Geometry: final body of the model. Coordinates: model frame, mm. Face numbers are marked on the shaded views. A direction names the side the tool comes from. Give positions to 0.01 mm unless a question says otherwise; leave off trailing zeros. Loops run counter-clockwise (first coordinate to the right, second up) from the corner with the lowest first, then second, coordinate; pieces in that order, holes last.
1. Section D-D, the plane x = -17.5. Output: boundary loops of the cut face in (y, z).
2. First-contact query: P1, Ø10, axis at y = -7.5, z = 57, coming from the +X side (3 decimals); P2, Ø2, axis at x = 8.5, z = -159.5, coming from the -Y side; P3, Ø10, axis at x = 20.5, z = 72, coming from the +Y side. Flat tips, straight axial feed; report the tip coordinate or a pass-through.
3. Section C-C, the plane x = 19. Output: boundary loops of the cut face in (y, z), then the cut area to 3 significant figures.
4. Access query for the marked faces 1, 2 and 3. Directions: +Z, -Z, +X, -X, +Y, -Y. A direction counts if a zero-diameter tool reaches every point of the face in a straight line with its end or side. Return the directions, or none.
5. Material intervals for line 1 along X through (y, z) = (-229.5, -87.5); line 2 along Z through (x, y) = (24, -132); line 3 along X through (y, z) = (-107, 112.5) (3 decimals), sorted ascending.
6. Draft query along Z for the marked faces 4 and 5. Return one class per face: +Z half, -Z half, draft (parallel to the pull), parting line (faces both ways), or undercut.
7. Section B-B, the plane y = 0. State how many separate pieces and enclosed holes the cut face has, then the cut area to 3 significant figures.
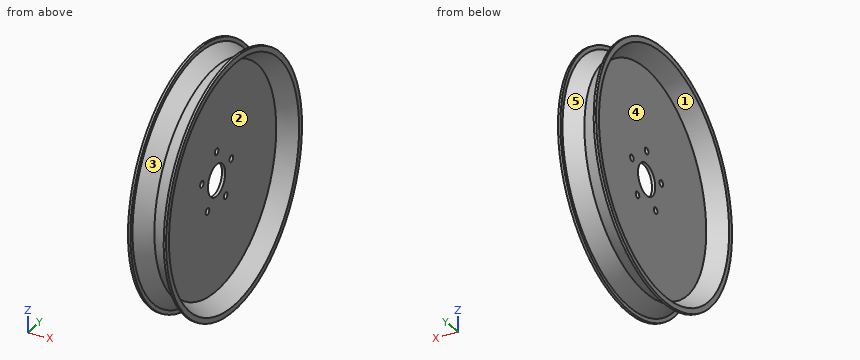
from build123d import *

# Parameters (mm, degrees)
F3_D = 13.1064


with BuildPart() as f1:
    # F0 (on Front) → F1 (revolve)
    with BuildSketch(Plane.XZ):
        Polygon((-3.175, 220.4975482247), (-3.175, 31.75), (3.175, 31.75), (3.175, 220.4975482247), (38.1, 240.6615063761), (38.1, 251.3486370331), (33.3375, 251.3486370331), (33.3375, 243.4111370331), (0, 224.163722434), (-33.3375, 243.4111370331), (-33.3375, 251.3486370331), (-38.1, 251.3486370331), (-38.1, 240.6615063761), align=None)
    revolve(axis=Axis((42.5242893398, 0, 0), (1, 0, 0)))

    # F3 (through all)
    with Locations(Plane.YZ.offset(3.175)):
        with Locations((0, 57.15), (54.3528799063, 17.6603212285), (33.5919271685, -46.2353212285), (-33.5919271685, -46.2353212285), (-54.3528799063, 17.6603212285)):
            Hole(F3_D / 2)


solid = f1.part
Answers below:
1. outline: circle Ø468.53 at (0, 0); hole circle Ø457.54 at (0, 0)
2. P1: stops at x = 3.175
2. P2: stops at y = -165.67
2. P3: stops at y = 228.15
3. outline: circle Ø470.27 at (0, 0); hole circle Ø459.27 at (0, 0)
3. area: 8,030 mm2
4. face 1: -X
4. face 2: +X
4. face 3: none
5. line 1: x = -38.1 to -33.34, 33.34 to 38.1
5. line 2: z = -198.06 to -191.42, 191.42 to 198.06
5. line 3: x = -3.175 to 3.175
6. face 4: undercut
6. face 5: parting line
7. separate pieces: 3
7. enclosed holes: 0
7. area: 3,270 mm2
